Verification items for this drawing (mm, ordinates from the low corner). A direction names the side the tool comes from. Give positions to 0.01 mm unless a question says otherwise; leave off trailing zeros. Loops run counter-clockwise (first coordinate to the right, second up) from the corner with the lowest first, then second, coordinate; pieces in that order, holes last. Notation, with made-up numbers: (11, 53) -> (39, 53) arc R15 ccw to (39, 58) -> close; hole circle Ø11 at (-13, 53). An arc over 180 degrees is marked (long way). Use one line per item in the form item = value. Start each with the question number.
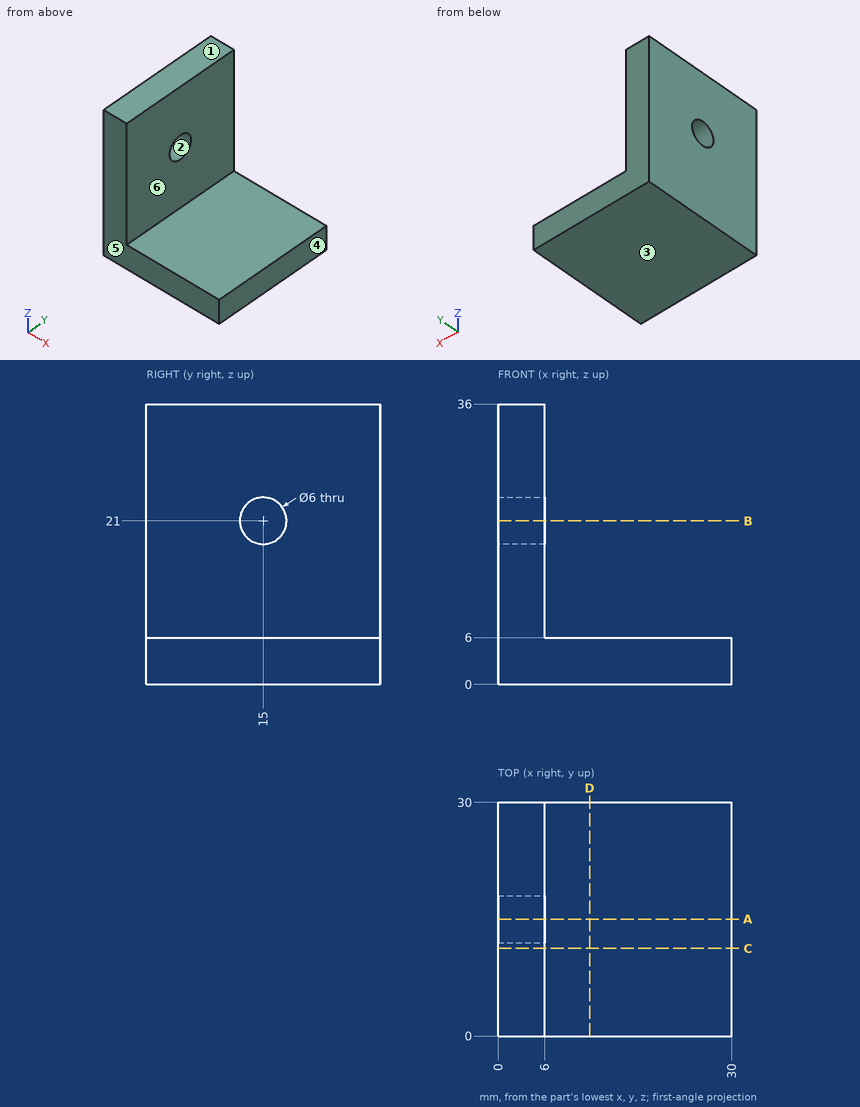
Item 1: Sectioned sample at C-C, the plane y = 11.25. Enter the section's corners in (x, z), and give its area (3 significant figures).
Item 2: Draft check along Z on the marked faces 1, 2, 3 and 4. Enter one of: +Z half, -Z half, draft (parallel to the pull), parting line (faces both ways), or undercut.
Item 3: Material ranges on line 1 (Y direction, x = 2, z = 21); line 2 (Z direction, x = 27, y = 2.5), recorded low to high.
Item 4: Gauge pin test, flat ends, axial feed: pin 1 Ø5 at (x, y) = (27, 5.5) entering from +Z; pin 2 Ø10 at (y, z) = (26.5, 32) entering from +X. Record the tip position at first contact, or that the pin passes through.
Item 5: Sectioned sample at B-B, the plane z = 21. Enter the section's corners in (x, y), and give its area (3 significant figures).
Item 6: Sectioned sample at A-A, the plane y = 15. Enter the section's corners in (x, z).
Item 7: Sectioned sample at D-D, the plane x = 11.75. Enter the section's corners in (y, z).
Item 8: Tool access check on the marked faces 5 and 6. Record the directions out of +Z, -Z, +X, -X, +Y, -Y that give a thin tool (end or side, any length) a straight path to the whole face; none if there is none.
Outcome:
q1.outline = (0, 0) -> (30, 0) -> (30, 6) -> (6, 6) -> (6, 36) -> (0, 36) -> close
q1.area = 360 mm^2
q2.face_1 = +Z half
q2.face_2 = undercut
q2.face_3 = -Z half
q2.face_4 = draft
q3.line_1 = 0 to 12, 18 to 30
q3.line_2 = 0 to 6
q4.pin_1 = 6
q4.pin_2 = 6
q5.outline = (0, 0) -> (6, 0) -> (6, 12) -> (0, 12) -> close; (0, 18) -> (6, 18) -> (6, 30) -> (0, 30) -> close
q5.area = 144 mm^2
q6.outline = (0, 0) -> (30, 0) -> (30, 6) -> (6, 6) -> (6, 18) -> (0, 18) -> close; (0, 24) -> (6, 24) -> (6, 36) -> (0, 36) -> close
q7.outline = (0, 0) -> (30, 0) -> (30, 6) -> (0, 6) -> close
q8.face_5 = +Z, -Z, +X, -X, -Y
q8.face_6 = +Z, +X, +Y, -Y
